Model file for the job. Use its own axes, mm. A direction names the side the tool comes from. Give positions to 0.01 mm unless a question says otherwise; leave off trailing zeros. Loops run counter-clockwise (first coordinate to the right, second up) from the corner with the lowest first, then second, coordinate; pieces in that order, holes last. Notation, with made-up numbers: (77.5, 62.5) - (109.5, 62.5) arc R32 ccw to (109.5, 94.5) - close; hole circle Ø9 at (-13, -19). An arc over 180 degrees is marked (long way). Use a Markdown table: item, result.
from build123d import *

# Parameters (mm, degrees)
BOSS_EXTRUDE5_DEPTH = 203.2
CUT_EXTRUDE3_START  = 9.525
CUT_EXTRUDE3_DEPTH  = 182.88


with BuildPart() as part:
    # Sketch6 → Boss-Extrude5 (new body)
    with BuildSketch(Plane(origin=(0, 0, 0), x_dir=(0, 0, -1), z_dir=(1, 0, 0))):
        Polygon((0, 0), (114.3, 0), (112.52602491, 50.8), (1.77397509, 50.8), align=None)
    extrude(amount=BOSS_EXTRUDE5_DEPTH)

    # Sketch9 → Cut-Extrude3 (cut)
    with BuildSketch(Plane(origin=(0, 0, 0), x_dir=(0, 0, -1), z_dir=(1, 0, 0)).offset(CUT_EXTRUDE3_START)):
        Polygon((103.847668826, 9.525), (102.738934394, 41.275), (10.97216067, 41.275), (9.863426239, 9.525), align=None)
    extrude(amount=CUT_EXTRUDE3_DEPTH, mode=Mode.SUBTRACT)


solid = part.part
(1) 3-axis set-ups, long thin cutter, end or side, ignore diameter. For faces 3 (the flat face through (203.2, 26, -56)), 4 (the flat face through (9.525, 26, -56)): which of +Z, -Z, +X, -X, +Y, -Y reach the whole face in a straight line?
Computed:
| item | result |
|---|---|
| face 3 | +Z, -Z, +X, +Y, -Y |
| face 4 | none |
(2) Slice it at A-A, the plane x = 110. Write the cut outline in (y, z) (3 decimals).
Computed:
| item | result |
|---|---|
| outline | (0, -114.3) - (50.8, -112.526) - (50.8, -1.774) - (0, 0) - close; hole (9.525, -103.848) - (41.275, -102.739) - (41.275, -10.972) - (9.525, -9.863) - close |
(3) Drill centre lines: probe 1 along X at (y, z) = (32, -98) (3 decimals); probe 2 along Y at (x, z) = (61, -86) (3 decimals); probe 3 along Z at (x, y) = (115, 19). Where is each one in solid material? Low to high. Write a range as [from, to].
Computed:
| item | result |
|---|---|
| probe 1 | [0, 9.525], [192.405, 203.2] |
| probe 2 | [0, 9.525], [41.275, 50.8] |
| probe 3 | [-113.64, -103.52], [-10.19, -0.66] |
(4) Pin check, flat tips, straight feed: P1, Ø10, axis at y = 35, z = -100, coming from the -X side; P2, Ø3, axis at x = 98.5, y = 20.5, coming from the +Z side; P3, Ø6, axis at x = 130.5, y = 42.5, coming from the +Z side; P4, Ø8, axis at x = 95.5, y = 31.5, coming from the -Z side. Stop position of each tip, or through.
Computed:
| item | result |
|---|---|
| P1 | x = 0 |
| P2 | z = -0.66 |
| P3 | z = -1.38 |
| P4 | z = -113.34 |
(5) Slice it at B-B, the plane z = -33. Write the cut outline in (x, y) (3 decimals).
Computed:
| item | result |
|---|---|
| outline | (0, 0) - (203.2, 0) - (203.2, 50.8) - (0, 50.8) - close; hole (9.525, 9.525) - (192.405, 9.525) - (192.405, 41.275) - (9.525, 41.275) - close |
(6) Mould opens along Z. For faces 1 (the flat face through (192.405, 26, -56)), 2 (the flat face through (0, 26, -56)) say: pulls with the +Z half, pulls with the -Z half, needs draft (parallel to the pull), parting line crosses it, or undercut.
Computed:
| item | result |
|---|---|
| face 1 | undercut |
| face 2 | needs draft |
